The listing builds one solid part. Answer for the finished solid, in the listing's coordinates (mm). Give positions to 0.01 mm unless a question says otherwise; leave off trailing zeros. Order: outer loops, then holes, each group sorted by start corner. A loop starts at its lowest first (then second) coordinate and runs counter-clockwise, first axis right, second up. Notation, with made-up numbers: (38, 44.25) - (52, 44.25) arc R17 cw to (52, 77.25) - close; hole circle Ø6 at (-34.5, 26.5). An arc over 180 degrees is marked (long way). Use CSV: the item, a comma, the result in double quotes.
```python
from build123d import *

# Parameters (mm, degrees)
SKETCH2_W           = 200
SKETCH2_H           = 20
BOSS_EXTRUDE1_DEPTH = 3
SKETCH3_R           = 5
CUT_EXTRUDE1_DEPTH  = 202.019899512
SKETCH4_R           = 5
CUT_EXTRUDE2_DEPTH  = 202.019899512
FILLET1_R           = 10
FILLET2_R           = 10
SKETCH5_R           = 5
CUT_EXTRUDE3_DEPTH  = 202.019899512


with BuildPart() as part:
    # Sketch2 → Boss-Extrude1 (new body)
    with BuildSketch(Plane(origin=(0, 0, 0), x_dir=(1, 0, 0), z_dir=(0, 1, 0))):
        with Locations((100, 10)):
            Rectangle(SKETCH2_W, SKETCH2_H)
    extrude(amount=BOSS_EXTRUDE1_DEPTH)

    # Sketch3 → Cut-Extrude1 (cut, through all)
    with BuildSketch(Plane(origin=(0, 3, 0), x_dir=(1, 0, 0), z_dir=(0, 1, 0))):
        with Locations(Location((9, 10, 0), (0, 0, 270))):
            Circle(SKETCH3_R)
    extrude(amount=-CUT_EXTRUDE1_DEPTH, mode=Mode.SUBTRACT)

    # Sketch4 → Cut-Extrude2 (cut, through all)
    with BuildSketch(Plane(origin=(0, 3, 0), x_dir=(1, 0, 0), z_dir=(0, 1, 0))):
        with Locations(Location((191, 10, 0), (0, 0, 270))):
            Circle(SKETCH4_R)
    extrude(amount=-CUT_EXTRUDE2_DEPTH, mode=Mode.SUBTRACT)

    # Fillet1
    fillet1_edges = [part.edges().sort_by_distance(p)[0] for p in [
        (0, 1.5, -20),
        (0, 1.5, 0),
    ]]
    fillet(fillet1_edges, radius=FILLET1_R - 0.0001)  # a hair under: the kernel refuses the full size

    # Fillet2
    fillet2_edges = [part.edges().sort_by_distance(p)[0] for p in [
        (200, 1.5, -20),
        (200, 1.5, 0),
    ]]
    fillet(fillet2_edges, radius=FILLET2_R - 0.0001)  # a hair under: the kernel refuses the full size

    # Sketch5 → Cut-Extrude3 (cut, through all)
    with BuildSketch(Plane(origin=(0, 3, 0), x_dir=(1, 0, 0), z_dir=(0, 1, 0))):
        with Locations(Location((135, 10, 0), (0, 0, 270))):
            Circle(SKETCH5_R)
    extrude(amount=-CUT_EXTRUDE3_DEPTH, mode=Mode.SUBTRACT)


solid = part.part
```
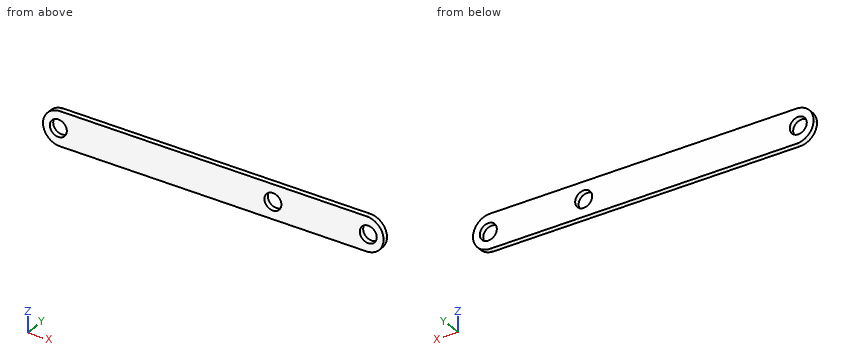
Item 1: Find the intervals of material crossed by line 1 along X through (y, z) = (0.6, -10.5); line 2 along X through (y, z) = (0.5, -12.25); line 3 along X through (y, z) = (0.1, -18.75), in increasing order.
Taken from the geometry:
line 1,"0.01 to 4.03, 13.97 to 130.03, 139.97 to 186.03, 195.97 to 199.99"
line 2,"0.26 to 4.53, 13.47 to 130.53, 139.47 to 186.53, 195.47 to 199.74"
line 3,"5.16 to 194.84"
Item 2: The part is cut by section B-B (x = 135). Give the vertices of the cut face in (y, z).
Taken from the geometry:
outline,"(0, -20) - (3, -20) - (3, -15) - (0, -15) - close; (0, -5) - (3, -5) - (3, 0) - (0, 0) - close"
Item 3: The part is cut by section C-C (z = -12.25). Give the vertices of the cut face in (x, y), and give its area (3 significant figures).
Taken from the geometry:
outline,"(0.26, 0) - (4.53, 0) - (4.53, 3) - (0.26, 3) - close; (13.47, 0) - (130.53, 0) - (130.53, 3) - (13.47, 3) - close; (139.47, 0) - (186.53, 0) - (186.53, 3) - (139.47, 3) - close; (195.47, 0) - (199.74, 0) - (199.74, 3) - (195.47, 3) - close"
area,"518 mm^2"
Item 4: The part is cut by section A-A (y = 1.9). Count the separate pieces of the cut face and the enclosed holes in it, and give its area (3 significant figures).
Taken from the geometry:
separate pieces,"1"
enclosed holes,"3"
area,"3,680 mm^2"
